```python
from build123d import *

# Parameters (mm, degrees)
SKETCH013_W          = 32
SKETCH013_H          = 3
POCKET_DEPTH         = 6.001
POCKET_DEPTH_BACK    = -6.001
POCKET001_DEPTH      = 6.001
POCKET001_DEPTH_BACK = -6.001
POCKET002_DEPTH      = 6.001
POCKET002_DEPTH_BACK = -6.001


with BuildPart() as part:
    # AdditivePipe: sweep along a path in Sketch002
    with BuildLine(Plane.XY) as additivepipe_path:
        ThreePointArc((0, 0), (-10.865453, 68.601773), (-42.398227, 130.488326))
    # Sketch → AdditivePipe (sweep)
    with BuildSketch(Plane.XZ):
        Polygon((-20, 6), (-20, -6), (-16, -6), (-16, -3), (-9, -3), (9, -3), (16, -3), (16, -6), (20, -6), (20, 6), (16, 6), (16, 3), (9, 3), (-9, 3), (-16, 3), (-16, 6), align=None)
    sweep(path=additivepipe_path.line)

    # AdditivePipe001: sweep along a path in Sketch001
    with BuildLine(Plane.XY) as additivepipe001_path:
        Line((0, 0), (0, 144))
    # Sketch → AdditivePipe001 (sweep)
    with BuildSketch(Plane.XZ):
        Polygon((-20, 6), (-20, -6), (-16, -6), (-16, -3), (-9, -3), (9, -3), (16, -3), (16, -6), (20, -6), (20, 6), (16, 6), (16, 3), (9, 3), (-9, 3), (-16, 3), (-16, 6), align=None)
    sweep(path=additivepipe001_path.line)

    # SubtractivePipe: sweep along a path in Sketch002
    with BuildLine(Plane.XY) as subtractivepipe_path:
        ThreePointArc((0, 0), (-10.865453, 68.601773), (-42.398227, 130.488326))
    # Sketch013 (on Face1 of AdditivePipe001) → SubtractivePipe (sweep, cut)
    with BuildSketch(Plane.XZ):
        with Locations((0, 4.5)):
            Rectangle(SKETCH013_W, SKETCH013_H)
    subtractivepipe = sweep(path=subtractivepipe_path.line, mode=Mode.SUBTRACT)

    # SubtractivePipe001: sweep along a path in Sketch001
    with BuildLine(Plane.XY) as subtractivepipe001_path:
        Line((0, 0), (0, 144))
    # Sketch013 (on Face1 of AdditivePipe001) → SubtractivePipe001 (sweep, cut)
    with BuildSketch(Plane.XZ):
        with Locations((0, 4.5)):
            Rectangle(SKETCH013_W, SKETCH013_H)
    subtractivepipe001 = sweep(path=subtractivepipe001_path.line, mode=Mode.SUBTRACT)

    # Mirrored: SubtractivePipe across XY
    add(subtractivepipe.mirror(Plane.XY), mode=Mode.SUBTRACT)

    # Mirrored001: SubtractivePipe001 across XY
    add(subtractivepipe001.mirror(Plane.XY), mode=Mode.SUBTRACT)

    # Sketch014 → Pocket (cut, two sides)
    with BuildSketch(Plane.XY) as pocket_sk:
        with BuildLine():
            Line((-4.5, 0), (4.5, 0))
            Line((4.5, 0), (4.5, 7))
            ThreePointArc((4.5, 7), (0, 19.361903), (-4.5, 7))
            Line((-4.5, 0), (-4.5, 7))
        make_face()
    extrude(amount=-POCKET_DEPTH, mode=Mode.SUBTRACT)
    extrude(pocket_sk.sketch, amount=-POCKET_DEPTH_BACK, mode=Mode.SUBTRACT)

    # Sketch015 → Pocket001 (cut, two sides)
    with BuildSketch(Plane.XY) as pocket001_sk:
        with BuildLine():
            Line((-46.038804, 127.843292), (-38.757651, 133.13336))
            Line((-38.757651, 133.13336), (-34.643154, 127.470241))
            ThreePointArc((-41.924307, 122.180173), (-31.017586, 114.824218), (-34.643154, 127.470241))
            Line((-46.038804, 127.843292), (-41.924307, 122.180173))
        make_face()
    extrude(amount=-POCKET001_DEPTH, mode=Mode.SUBTRACT)
    extrude(pocket001_sk.sketch, amount=-POCKET001_DEPTH_BACK, mode=Mode.SUBTRACT)

    # Sketch016 → Pocket002 (cut, two sides)
    with BuildSketch(Plane.XY) as pocket002_sk:
        with BuildLine():
            Line((-4.5, 144), (4.5, 144))
            Line((4.5, 144), (4.5, 137))
            ThreePointArc((-4.5, 137), (0, 124.638097), (4.5, 137))
            Line((-4.5, 144), (-4.5, 137))
        make_face()
    extrude(amount=-POCKET002_DEPTH, mode=Mode.SUBTRACT)
    extrude(pocket002_sk.sketch, amount=-POCKET002_DEPTH_BACK, mode=Mode.SUBTRACT)


solid = part.part
```
Work out the finished part from the listing and answer in its coordinate system (mm). A direction names the side the tool comes from. Give positions to 0.01 mm unless a question says otherwise; leave off trailing zeros. Order: outer loops, then holes, each group sorted by start corner. A loop starts at its lowest first (then second) coordinate and runs counter-clockwise, first axis right, second up. Notation, with made-up numbers: (71.5, -10) -> (88.5, -10) arc R22 cw to (88.5, 5) -> close; hole circle Ø3 at (52, 16). An arc over 180 degrees is marked (long way). Answer as CSV lines item,"result". Start each with the question number.
(1) Section D-D, the plane x = -23 is taken. Write down the section's boundary in (y, z).
(2) For a pull along Z with two mould halves and no side action, classify faces 1 (the cylindrical face through (-22.36, 129.57, 4.48)), 2 (the flat face through (17, 77, -6)), 3 (the flat face through (-19, 134, 6)) as released by +Z, released by -Z, zero draft, split by the parting line, or undercut.
(3) Consider line 1 along Y through (x, z) = (6, 2.5); line 2 along Y through (x, z) = (0, -0.75); line 3 along Z through (x, y) = (-50, 114). Determine where each line is inside the solid, lowest interval first.
(4) Section A-A, the plane x = -36 is taken. Write down the section's boundary in (y, z).
(5) Each of these flat-tipped pins is pushed along its axis until it touches: pin 1 Ø16 at (x, y) = (-35.13, 120.49) entering from +Z; pin 2 Ø0.9 at (y, z) = (101.5, -4) entering from -X; pin 3 Ø2.5 at (y, z) = (80.5, 4) entering from -X. Where does it stop, or does it pass through?
(6) Which of the six approach directions +Z, -Z, +X, -X, +Y, -Y give full straight-line access (tool end or side, diameter ignored) to faces 4 (the flat face through (4.5, 141, 0)), 5 (the flat face through (16, 73, -4)), 6 (the cylindrical face through (-25.804, 62.795, -4.479)), 7 (the flat face through (-4.5, 3, 0))?
(7) Section B-B, the plane z = 1 is taken. Write down the section's boundary in (x, y), plus the area to 3 significant figures.
(8) Section C-C, the plane y = 50.5 is taken. Write down the section's boundary in (x, z), plus the area to 3 significant figures.
Entries:
1,outline,"(34.68, -6) -> (53.24, -6) -> (53.24, -3) -> (130.55, -3) -> (130.55, -6) -> (137.71, -6) -> (137.71, 6) -> (130.55, 6) -> (130.55, 3) -> (53.24, 3) -> (53.24, 6) -> (34.68, 6) -> close"
2,face 1,"zero draft"
2,face 2,"released by -Z"
2,face 3,"released by +Z"
3,line 1,"0 to 8.76, 15.97 to 128.03, 135.24 to 144"
3,line 2,"19.36 to 124.64"
3,line 3,"-3 to 3"
4,outline,"(78.79, -6) -> (88.54, -6) -> (88.54, -3) -> (113.54, -3) -> (113.54, 3) -> (88.54, 3) -> (88.54, 6) -> (78.79, 6) -> close; (129.34, -3) -> (135.14, -3) -> (135.14, 3) -> (129.34, 3) -> close"
5,pin 1,"z = 3"
5,pin 2,"x = -47.61"
5,pin 3,"x = -37.28"
6,face 4,"+Z, -Z, +Y"
6,face 5,"-Z, +Y, -Y"
6,face 6,"-Z"
6,face 7,"+Z, -Z, -Y"
7,outline,"(-58.58, 118.73) arc R202 cw to (-20, 0) -> (-4.5, 0) -> (-4.5, 7) arc R7 cw (long way) to (4.5, 7) -> (4.5, 0) -> (20, 0) -> (20, 144) -> (4.5, 144) -> (4.5, 137) arc R7 cw (long way) to (-4.5, 137) -> (-4.5, 144) -> (-20, 144) -> (-20, 133.27) arc R242 ccw to (-26.22, 142.24) -> (-38.76, 133.13) -> (-34.64, 127.47) arc R7 cw (long way) to (-41.92, 122.18) -> (-46.04, 127.84) -> close"
7,area,"7,100 mm²"
8,outline,"(-26.41, -6) -> (-22.29, -6) -> (-22.29, -3) -> (16, -3) -> (16, -6) -> (20, -6) -> (20, 6) -> (16, 6) -> (16, 3) -> (-22.29, 3) -> (-22.29, 6) -> (-26.41, 6) -> close"
8,area,"327 mm²"
